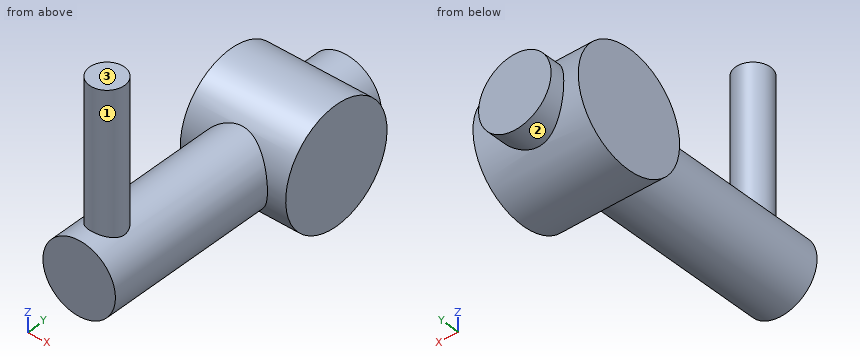
from build123d import *

# Parameters (mm, degrees)
CYLINDER012_R     = 2.5
CYLINDER012_DEPTH = 21
CYLINDER011_R     = 1.2
CYLINDER011_DEPTH = 12
CYLINDER010_R     = 4
CYLINDER010_DEPTH = 7.26


with BuildPart() as cylinder012:
    # Cylinder012 → Cylinder012 (new body)
    with BuildSketch(Plane(origin=(3.5, 5, 0), x_dir=(1, 0, 0), z_dir=(0, -1, 0))):
        Circle(CYLINDER012_R)
    extrude(amount=CYLINDER012_DEPTH)


with BuildPart() as cylinder011:
    # Cylinder011 → Cylinder011 (new body)
    with BuildSketch(Plane(origin=(3.5, -13.8, 0), x_dir=(1, 0, 0), z_dir=(0, 0, 1))):
        Circle(CYLINDER011_R)
    extrude(amount=CYLINDER011_DEPTH)


with BuildPart() as valve003:
    # Cylinder010 → Cylinder010 (new body)
    with BuildSketch(Plane(origin=(0, 0, 0), x_dir=(0, 0, -1), z_dir=(1, 0, 0))):
        Circle(CYLINDER010_R)
    extrude(amount=CYLINDER010_DEPTH)

    # Fusion003: union Cylinder012, Cylinder011
    add(cylinder012.part)
    add(cylinder011.part)


with BuildPart() as valve003_1:
    # Fusion003 placement: moved
    add(valve003.part.moved(Location((10, 0, 62.56))))


solid = valve003_1.part
Model file for the job. Use its own axes, mm. Face numbers are marked on the shaded views. A direction names the side the tool comes from. Round coordinates to 2 decimals unless told otherwise and drop trailing zeros. Loops run counter-clockwise (first coordinate to the right, second up) from the corner with the lowest first, then second, coordinate; pieces in that order, holes last.
1. Band-saw the part on A-A, the plane z = 62.56. List the corners of the cut face in (x, y).
Check values:
outline: (10, -4) - (11, -4) - (11, -16) - (16, -16) - (16, -4) - (17.26, -4) - (17.26, 4) - (16, 4) - (16, 5) - (11, 5) - (11, 4) - (10, 4) - close
2. Band-saw the part on C-C, the plane y = -13.8. List the corners of the cut face in (x, z), and give its area (3 significant figures).
Check values:
outline: (12.3, 64.75) arc R2.5 ccw (long way) to (14.7, 64.75) - (14.7, 74.56) - (12.3, 74.56) - close
area: 42.7 mm2
3. Drop flat-ended pins along their axis: P1, Ø1.5, axis at x = 15, y = -2.5, coming from the -Z side; P2, Ø1, axis at x = 12.5, z = 71.5, coming from the +Y side. Give the stop position or say it passes through.
Check values:
P1: stops at z = 58.96
P2: stops at y = -12.71
4. Tool access for the marked faces 1, 2 and 3: list every direction of +Z, -Z, +X, -X, +Y, -Y with a clear straight run to the whole face (end or side of a thin tool).
Check values:
face 1: +Z
face 2: +Y
face 3: +Z, +X, -X, +Y, -Y
5. Band-saw the part on B-B, the plane x = 13.5. List the corners of the cut face in (y, z).
Check values:
outline: (-16, 60.06) - (-3.12, 60.06) arc R4 ccw to (3.12, 60.06) - (5, 60.06) - (5, 65.06) - (3.12, 65.06) arc R4 ccw to (-3.12, 65.06) - (-12.6, 65.06) - (-12.6, 74.56) - (-15, 74.56) - (-15, 65.06) - (-16, 65.06) - close
6. Band-saw the part on D-D, the plane x = 11.5. List the corners of the cut face in (y, z), and give its area (3 significant figures).
Check values:
outline: (-16, 61.06) - (-3.71, 61.06) arc R4 ccw to (3.71, 61.06) - (5, 61.06) - (5, 64.06) - (3.71, 64.06) arc R4 ccw to (-3.71, 64.06) - (-16, 64.06) - close
area: 89.8 mm2
7. Wall check: probe 1 along X at (y, z) = (-9.75, 64.75); probe 2 along Z at (x, y) = (15, -14.5); probe 3 along Y at (x, z) = (14, 65.75). Give the ranges that are in metal, low to high.
Check values:
probe 1: x = 12.29 to 14.71
probe 2: z = 60.56 to 64.56
probe 3: y = -14.89 to -12.71, -2.41 to 2.41
